from build123d import *

# Parameters (mm, degrees)
SKETCH3_W                     = 100
SKETCH3_H                     = 79
BOSS_EXTRUDE1_DEPTH           = 3.175
SKETCH5_W                     = 58.8
SKETCH5_H                     = 40
CUT_EXTRUDE2_DEPTH            = 3.175
SKETCH11_W                    = 6.35
SKETCH11_H                    = 3.175
BOSS_EXTRUDE2_DEPTH           = 3.175
LPATTERN2_COUNT               = 6
LPATTERN2_PITCH               = 6.35
LPATTERN2_COPY_1_SKETCH_W     = 6.35
LPATTERN2_COPY_1_SKETCH_H     = 3.175
LPATTERN2_COPY_1_DEPTH        = 3.175
LPATTERN2_COPY_2_SKETCH_W     = 6.35
LPATTERN2_COPY_2_SKETCH_H     = 3.175
LPATTERN2_COPY_2_DEPTH        = 3.175
LPATTERN2_COPY_3_SKETCH_W     = 6.35
LPATTERN2_COPY_3_SKETCH_H     = 3.175
LPATTERN2_COPY_3_DEPTH        = 3.175
LPATTERN2_COPY_4_SKETCH_W     = 6.35
LPATTERN2_COPY_4_SKETCH_H     = 3.175
LPATTERN2_COPY_4_DEPTH        = 3.175
LPATTERN2_COPY_5_SKETCH_W     = 6.35
LPATTERN2_COPY_5_SKETCH_H     = 3.175
LPATTERN2_COPY_5_DEPTH        = 3.175
LPATTERN2_COL_COUNT           = 6
LPATTERN2_COL_PITCH           = 6.35
LPATTERN2_COL_COPY_1_SKETCH_W = 6.35
LPATTERN2_COL_COPY_1_SKETCH_H = 3.175
LPATTERN2_COL_COPY_1_DEPTH    = 3.175
LPATTERN2_COL_COPY_2_SKETCH_W = 6.35
LPATTERN2_COL_COPY_2_SKETCH_H = 3.175
LPATTERN2_COL_COPY_2_DEPTH    = 3.175
LPATTERN2_COL_COPY_3_SKETCH_W = 6.35
LPATTERN2_COL_COPY_3_SKETCH_H = 3.175
LPATTERN2_COL_COPY_3_DEPTH    = 3.175
LPATTERN2_COL_COPY_4_SKETCH_W = 6.35
LPATTERN2_COL_COPY_4_SKETCH_H = 3.175
LPATTERN2_COL_COPY_4_DEPTH    = 3.175
LPATTERN2_COL_COPY_5_SKETCH_W = 6.35
LPATTERN2_COL_COPY_5_SKETCH_H = 3.175
LPATTERN2_COL_COPY_5_DEPTH    = 3.175
SKETCH13_W                    = 12.35
SKETCH13_H                    = 79
BOSS_EXTRUDE4_DEPTH           = 3.175
SKETCH14_W                    = 12.35
SKETCH14_H                    = 79
BOSS_EXTRUDE5_DEPTH           = 3.175
SKETCH15_R                    = 1.5
CUT_EXTRUDE4_DEPTH            = 10
SKETCH16_R                    = 1.5
CUT_EXTRUDE5_DEPTH            = 10
SKETCH17_W                    = 12.35
SKETCH17_H                    = 79
CUT_EXTRUDE6_DEPTH            = 10


with BuildPart() as part:
    # Sketch3 → Boss-Extrude1 (new body)
    with BuildSketch(Plane(origin=(0, 0, 0), x_dir=(1, 0, 0), z_dir=(0, 1, 0))):
        with Locations((46, 22.5)):
            Rectangle(SKETCH3_W, SKETCH3_H)
    extrude(amount=BOSS_EXTRUDE1_DEPTH)

    # Sketch5 → Cut-Extrude2 (cut)
    with BuildSketch(Plane(origin=(0, 3.175, 0), x_dir=(1, 0, 0), z_dir=(0, 1, 0))):
        with Locations((44, 42)):
            Rectangle(SKETCH5_W, SKETCH5_H)
    extrude(amount=-CUT_EXTRUDE2_DEPTH, mode=Mode.SUBTRACT)

    # Sketch11 → Boss-Extrude2 (add)
    with BuildSketch(Plane(origin=(0, 3.175, 0), x_dir=(1, 0, 0), z_dir=(0, 1, 0))):
        with Locations((-4, 22.5)):
            Rectangle(SKETCH11_W, SKETCH11_H)
    boss_extrude2 = extrude(amount=-BOSS_EXTRUDE2_DEPTH)

    # Mirror2: Boss-Extrude2 across plane
    add(boss_extrude2.mirror(Plane.ZY.offset(-46)))

    # LPattern2: Boss-Extrude2 ×6
    with Locations(*[(0, 0, -i * LPATTERN2_PITCH) for i in range(1, LPATTERN2_COUNT)]):
        add(boss_extrude2)

    # LPattern2 copy 1 sketch → LPattern2 copy 1 (add)
    with BuildSketch(Plane(origin=(92, 3.175, -6.35), x_dir=(-1, 0, 0), z_dir=(0, 1, 0))):
        with Locations((-4, -22.5)):
            Rectangle(LPATTERN2_COPY_1_SKETCH_W, LPATTERN2_COPY_1_SKETCH_H)
    extrude(amount=-LPATTERN2_COPY_1_DEPTH)

    # LPattern2 copy 2 sketch → LPattern2 copy 2 (add)
    with BuildSketch(Plane(origin=(92, 3.175, -12.7), x_dir=(-1, 0, 0), z_dir=(0, 1, 0))):
        with Locations((-4, -22.5)):
            Rectangle(LPATTERN2_COPY_2_SKETCH_W, LPATTERN2_COPY_2_SKETCH_H)
    extrude(amount=-LPATTERN2_COPY_2_DEPTH)

    # LPattern2 copy 3 sketch → LPattern2 copy 3 (add)
    with BuildSketch(Plane(origin=(92, 3.175, -19.05), x_dir=(-1, 0, 0), z_dir=(0, 1, 0))):
        with Locations((-4, -22.5)):
            Rectangle(LPATTERN2_COPY_3_SKETCH_W, LPATTERN2_COPY_3_SKETCH_H)
    extrude(amount=-LPATTERN2_COPY_3_DEPTH)

    # LPattern2 copy 4 sketch → LPattern2 copy 4 (add)
    with BuildSketch(Plane(origin=(92, 3.175, -25.4), x_dir=(-1, 0, 0), z_dir=(0, 1, 0))):
        with Locations((-4, -22.5)):
            Rectangle(LPATTERN2_COPY_4_SKETCH_W, LPATTERN2_COPY_4_SKETCH_H)
    extrude(amount=-LPATTERN2_COPY_4_DEPTH)

    # LPattern2 copy 5 sketch → LPattern2 copy 5 (add)
    with BuildSketch(Plane(origin=(92, 3.175, -31.75), x_dir=(-1, 0, 0), z_dir=(0, 1, 0))):
        with Locations((-4, -22.5)):
            Rectangle(LPATTERN2_COPY_5_SKETCH_W, LPATTERN2_COPY_5_SKETCH_H)
    extrude(amount=-LPATTERN2_COPY_5_DEPTH)

    # LPattern2 col: Boss-Extrude2 ×6
    with Locations(*[(0, 0, i * LPATTERN2_COL_PITCH) for i in range(1, LPATTERN2_COL_COUNT)]):
        add(boss_extrude2)

    # LPattern2 col copy 1 sketch → LPattern2 col copy 1 (add)
    with BuildSketch(Plane(origin=(92, 3.175, 6.35), x_dir=(-1, 0, 0), z_dir=(0, 1, 0))):
        with Locations((-4, -22.5)):
            Rectangle(LPATTERN2_COL_COPY_1_SKETCH_W, LPATTERN2_COL_COPY_1_SKETCH_H)
    extrude(amount=-LPATTERN2_COL_COPY_1_DEPTH)

    # LPattern2 col copy 2 sketch → LPattern2 col copy 2 (add)
    with BuildSketch(Plane(origin=(92, 3.175, 12.7), x_dir=(-1, 0, 0), z_dir=(0, 1, 0))):
        with Locations((-4, -22.5)):
            Rectangle(LPATTERN2_COL_COPY_2_SKETCH_W, LPATTERN2_COL_COPY_2_SKETCH_H)
    extrude(amount=-LPATTERN2_COL_COPY_2_DEPTH)

    # LPattern2 col copy 3 sketch → LPattern2 col copy 3 (add)
    with BuildSketch(Plane(origin=(92, 3.175, 19.05), x_dir=(-1, 0, 0), z_dir=(0, 1, 0))):
        with Locations((-4, -22.5)):
            Rectangle(LPATTERN2_COL_COPY_3_SKETCH_W, LPATTERN2_COL_COPY_3_SKETCH_H)
    extrude(amount=-LPATTERN2_COL_COPY_3_DEPTH)

    # LPattern2 col copy 4 sketch → LPattern2 col copy 4 (add)
    with BuildSketch(Plane(origin=(92, 3.175, 25.4), x_dir=(-1, 0, 0), z_dir=(0, 1, 0))):
        with Locations((-4, -22.5)):
            Rectangle(LPATTERN2_COL_COPY_4_SKETCH_W, LPATTERN2_COL_COPY_4_SKETCH_H)
    extrude(amount=-LPATTERN2_COL_COPY_4_DEPTH)

    # LPattern2 col copy 5 sketch → LPattern2 col copy 5 (add)
    with BuildSketch(Plane(origin=(92, 3.175, 31.75), x_dir=(-1, 0, 0), z_dir=(0, 1, 0))):
        with Locations((-4, -22.5)):
            Rectangle(LPATTERN2_COL_COPY_5_SKETCH_W, LPATTERN2_COL_COPY_5_SKETCH_H)
    extrude(amount=-LPATTERN2_COL_COPY_5_DEPTH)

    # Sketch13 → Boss-Extrude4 (add)
    with BuildSketch(Plane(origin=(0, 3.175, 0), x_dir=(1, 0, 0), z_dir=(0, 1, 0))):
        with Locations((-13.35, 22.5)):
            Rectangle(SKETCH13_W, SKETCH13_H)
    extrude(amount=-BOSS_EXTRUDE4_DEPTH)

    # Sketch14 → Boss-Extrude5 (add)
    with BuildSketch(Plane(origin=(0, 3.175, 0), x_dir=(1, 0, 0), z_dir=(0, 1, 0))):
        with Locations((105.35, 22.5)):
            Rectangle(SKETCH14_W, SKETCH14_H)
    extrude(amount=-BOSS_EXTRUDE5_DEPTH)

    # Sketch15 → Cut-Extrude4 (cut)
    with BuildSketch(Plane(origin=(0, 3.175, 0), x_dir=(1, 0, 0), z_dir=(0, 1, 0))):
        with Locations(Location((-13.35, 54, 0), (0, 0, 270))):
            Circle(SKETCH15_R)
        with Locations(Location((-13.35, -9, 0), (0, 0, 270))):
            Circle(SKETCH15_R)
    extrude(amount=-CUT_EXTRUDE4_DEPTH, mode=Mode.SUBTRACT)

    # Sketch16 → Cut-Extrude5 (cut)
    with BuildSketch(Plane(origin=(0, 3.175, 0), x_dir=(1, 0, 0), z_dir=(0, 1, 0))):
        with Locations(Location((105.35, 54, 0), (0, 0, 270))):
            Circle(SKETCH16_R)
        with Locations(Location((105.35, -9, 0), (0, 0, 270))):
            Circle(SKETCH16_R)
    extrude(amount=-CUT_EXTRUDE5_DEPTH, mode=Mode.SUBTRACT)

    # Sketch17 → Cut-Extrude6 (cut)
    with BuildSketch(Plane(origin=(0, 3.175, 0), x_dir=(1, 0, 0), z_dir=(0, 1, 0))):
        with Locations((-13.35, 22.5)):
            Rectangle(SKETCH17_W, SKETCH17_H)
        with Locations((105.35, 22.5)):
            Rectangle(SKETCH17_W, SKETCH17_H)
    extrude(amount=-CUT_EXTRUDE6_DEPTH, mode=Mode.SUBTRACT)


solid = part.part
Here's how the part is built. I have some questions about the finished solid (model axes, mm). A direction names the side the tool comes from. Coordinates: 2 decimals unless noted, no trailing zeros. Order: outer loops, then holes, each group sorted by start corner. A loop starts at its lowest first (then second) coordinate and runs counter-clockwise, first axis right, second up. Notation, with made-up numbers: (63, 86) - (81, 86) arc R14 cw to (81, 108) - close; hole circle Ø6 at (-18.75, 77.5). An arc over 180 degrees is marked (long way). Use CSV: the item, a comma, the result in double quotes. Start each with the question number.
1. I'm going to push flat-ended pins straight in: pin 1 (1 mm diameter, centred on x = 98, y = 2, fed in from -Z); pin 2 (1.6 mm diameter, centred on y = 2.5, z = -13, fed in from -X). Where does each tip first touch, or does it pass through?
2. If we mould it in two halves opening along Z, with no side actions, what happens to faces 1 (the face through (5, 2, -62)), 2 (the face through (-6, 2, -27.263)), 3 (the face through (98, 2, 10.838)), 4 (the face through (-4, 2, 14))? For each: +Z half, -Z half, draft (parallel to the pull), parting line (faces both ways), or undercut.
3. Suppose I cut it at B-B on x = 35.5. List the corners of the cut face in (y, z) for me (3 decimals), then the cut area to 3 significant figures.
4. Suppose I cut it at A-A on z = 0. List the corners of the cut face in (x, y) for me (3 decimals).
5. For faces 5 (the face through (-4, 2, -38)), 6 (the face through (99.175, 2, -16)), 7 (the face through (14.6, 2, -42)), 8 (the face through (96, 2, -59)), 9 (the face through (98, 2, -27.263)), which set-ups out of +Z, -Z, +X, -X, +Y, -Y let a thin tool reach every point of the face, with its end or its side?
6. Please list where these lines run through material, in increasing order: line 1 (X direction, y = 3, z = -44); line 2 (X direction, y = 2.8, z = -36.5) (3 decimals); line 3 (Z direction, x = 56, y = 1.9). Write a range as from..to.
Output:
1,pin 1,"stops at z = -55.84"
1,pin 2,"stops at x = -4"
2,face 1,"-Z half"
2,face 2,"undercut"
2,face 3,"+Z half"
2,face 4,"draft"
3,outline,"(0, -22) - (3.175, -22) - (3.175, 17) - (0, 17) - close"
3,area,"124 mm2"
4,outline,"(-4, 0) - (96, 0) - (96, 3.175) - (-4, 3.175) - close"
5,face 5,"-X, +Y, -Y"
5,face 6,"+Z, -Z, +X, +Y, -Y"
5,face 7,"-Z, +Y, -Y"
5,face 8,"-Z, +X, +Y, -Y"
5,face 9,"+X, +Y, -Y"
6,line 1,"x = -4..14.6, 73.4..96"
6,line 2,"x = -7.175..14.6, 73.4..99.175"
6,line 3,"z = -22..17"
